```python
from build123d import *

# Parameters (mm, degrees)
SKETCH_1_R          = 17.35
EXTRUDE_1_DEPTH     = 5
CHAMFER_1_SIZE      = 2
SKETCH_2_R          = 4
CUT_EXTRUDE_1_DEPTH = 5
SKETCH_3_R          = 1.5
CUT_EXTRUDE_2_DEPTH = 5
CUT_EXTRUDE_3_DEPTH = 3.5


with BuildPart() as part:
    # 草图1 → 凸台-拉伸1 (new body)
    with BuildSketch(Plane(origin=(0, 0, 0), x_dir=(1, 0, 0), z_dir=(0, 1, 0))):
        with Locations(Location((0, 0, 0), (0, 0, 270))):
            Circle(SKETCH_1_R)
    extrude(amount=EXTRUDE_1_DEPTH)

    # 倒角1
    chamfer_1_edges = [part.edges().sort_by_distance(p)[0] for p in [
        (0, 0, -17.35),
    ]]
    chamfer(chamfer_1_edges, length=CHAMFER_1_SIZE)

    # 草图2 → 切除-拉伸1 (cut)
    with BuildSketch(Plane(origin=(0, 5, 0), x_dir=(1, 0, 0), z_dir=(0, 1, 0))):
        with Locations(Location((0, 0, 0), (0, 0, 270))):
            Circle(SKETCH_2_R)
    extrude(amount=-CUT_EXTRUDE_1_DEPTH, mode=Mode.SUBTRACT)

    # 草图3 → 切除-拉伸2 (cut)
    with BuildSketch(Plane.XZ):
        with Locations(Location((-6.75, 6.75, 0), (0, 0, 270))):
            Circle(SKETCH_3_R)
        with Locations(Location((6.75, 6.75, 0), (0, 0, 270))):
            Circle(SKETCH_3_R)
        with Locations(Location((6.75, -6.75, 0), (0, 0, 270))):
            Circle(SKETCH_3_R)
        with Locations(Location((-6.75, -6.75, 0), (0, 0, 270))):
            Circle(SKETCH_3_R)
    extrude(amount=-CUT_EXTRUDE_2_DEPTH, mode=Mode.SUBTRACT)

    # 草图4 → 切除-拉伸3 (cut)
    with BuildSketch(Plane.XZ):
        with BuildLine():
            Line((14.35, 3), (21.35, 3))
            Line((21.35, 3), (21.35, -3))
            Line((21.35, -3), (14.35, -3))
            ThreePointArc((14.35, -3), (13.642893219, -2.707106781), (13.35, -2))
            Line((13.35, -2), (13.35, 2))
            ThreePointArc((13.35, 2), (13.642893219, 2.707106781), (14.35, 3))
        make_face()
    extrude(amount=-CUT_EXTRUDE_3_DEPTH, mode=Mode.SUBTRACT)


solid = part.part
```
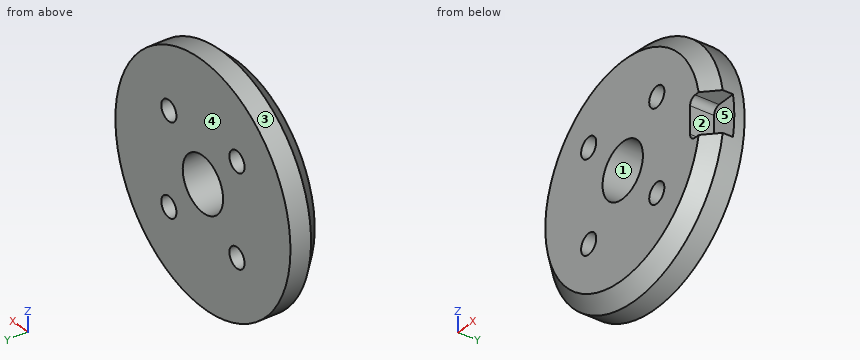
Verification items for the finished model (mm, model axes). Face numbers are marked on the shaded views. A direction names the side the tool comes from. Give positions to 0.01 mm unless a question says otherwise; leave off trailing zeros. Order: outer loops, then holes, each group sorted by start corner. A loop starts at its lowest first (then second) coordinate and runs counter-clockwise, first axis right, second up. Notation, with made-up numbers: M -34.75,76.25 L -12.75,76.25 A26 ccw -12.75,107.25 Z; hole C 44.5,55.5 d3. An arc over 180 degrees is marked long. Answer in a Markdown table with one row per item. Add a question column.
Item 1: Mould release check, pull along Z, two halves, no side actions. Record for the marked faces 3, 4 and 5: released by +Z, released by -Z, zero draft, split by the parting line, or undercut.
Item 2: Scan lines: probe 1 along X at (y, z) = (2.8, 0); probe 2 along X at (y, z) = (2, 6.75); probe 3 along X at (y, z) = (3.55, 0). Record each from-to range of solid material in increasing order. Write a range as from..to.
Item 3: Section check C-C, the plane x = -6.75. State how many separate pieces and enclosed holes the cut face has, and give its area (3 significant figures).
Item 4: Tool access check on the marked faces 1 and 2. Record the directions out of +Z, -Z, +X, -X, +Y, -Y that give a thin tool (end or side, any length) a straight path to the whole face; none if there is none.
Item 5: Gauge pin test, flat ends, axial feed: pin 1 (1.8 mm diameter, centred on y = 2.5, z = 0.5, fed in from +X); pin 2 (2 mm diameter, centred on x = 16.5, y = 2.5, fed in from +Z); pin 3 (1.5 mm diameter, centred on x = -11.5, z = 5.5, fed in from -Y); pin 4 (1.5 mm diameter, centred on y = 3, z = -9.5, fed in from +X). Record the tip position at first contact, or that the pin passes through.
Item 6: Section check B-B, the plane y = 2.9. Enter the section's corners in (x, z), and give its area (3 significant figures).
Item 7: Section check A-A, the plane z = 0. Enter the section's corners in (x, y).
Filled sheet:
| question | item | result |
|---|---|---|
| 1 | face 3 | split by the parting line |
| 1 | face 4 | zero draft |
| 1 | face 5 | undercut |
| 2 | probe 1 | x = -17.35..-4, 4..13.35 |
| 2 | probe 2 | x = -15.98..-8.25, -5.25..5.25, 8.25..15.98 |
| 2 | probe 3 | x = -17.35..-4, 4..17.35 |
| 3 | separate pieces | 3 |
| 3 | enclosed holes | 0 |
| 3 | area | 125 mm^2 |
| 4 | face 1 | +Y, -Y |
| 4 | face 2 | +X, -Y |
| 5 | pin 1 | stops at x = 13.35 |
| 5 | pin 2 | stops at z = 7.8 |
| 5 | pin 3 | stops at y = 0 |
| 5 | pin 4 | stops at x = 14.98 |
| 6 | outline | M 13.35,-2 L 13.35,2 A1 cw 14.35,3 L 17.09,3 A17.35 ccw long 17.09,-3 L 14.35,-3 A1 cw Z; hole C -6.75,-6.75 d3; hole C -6.75,6.75 d3; hole C 0,0 d8; hole C 6.75,-6.75 d3; hole C 6.75,6.75 d3 |
| 6 | area | 844 mm^2 |
| 7 | outline | M -17.35,2 L -15.35,0 L -4,0 L -4,5 L -17.35,5 Z; M 4,0 L 13.35,0 L 13.35,3.5 L 17.35,3.5 L 17.35,5 L 4,5 Z |
